Design review of the part built by this model. Coordinates are the model's own, in mm. A direction names the side the tool comes from. Coordinates: 2 decimals unless noted, no trailing zeros. Loops run counter-clockwise (first coordinate to the right, second up) from the corner with the lowest first, then second, coordinate; pieces in that order, holes last. Notation, with made-up numbers: (-5.75, -34) -> (3.25, -34) arc R15 cw to (3.25, -5) -> close; hole circle Ø1 at (71, -36). An arc over 180 degrees is marked (long way). One line per item, written item: value. Start each with the question number.
1. Add section B-B on x = 125.37. Write out the cut boundary in (y, z), plus the area to 3 significant figures.
2. Insertion check: pin 1 (4 mm diameter, centred on x = 7.86, z = 16.83, fed in from -Y). The pin has a flat end and moves straight along its axis. Give the tip position at first contact, or say it passes through.
3. Add section A-A on z = 16.83. Write out the cut boundary in (x, y).
4. Add section C-C on y = 1.15. Write out the cut boundary in (x, z).
5. Add section D-D on x = 80.5. Write out the cut boundary in (y, z).
6. Machinability: for faces 5 (the flat face through (92, 1, 21.85)), 6 (the flat face through (64, 0, 37)), which of the approach directions +Z, -Z, +X, -X, +Y, -Y give a long, thin tool a straight path to every point of the face, cutting with its end or side? Answer none if there is none.
7. For probe 1 along X at (y, z) = (1.4, 22.15); probe 2 along Z at (x, y) = (56.47, 1.25); probe 3 along Z at (x, y) = (95, 1.6), list the stretches that pass through material, from the lowest coordinate up.
8. Draft analysis for pull direction Z (two halves, no side actions). For faces 1 (the flat face through (64, 1, 75.8)), 2 (the flat face through (64, 3, 37)), 3 (the flat face through (119.47, 1, 38)), 4 (the cylindrical face through (8.87, 1.52, 15.72)), state which applies: pulls with the +Z half, pulls with the -Z half, needs draft (parallel to the pull), parting line crosses it, or undercut.
```python
from build123d import *

# Parameters (mm, degrees)
SKETCH1_W           = 130.41
SKETCH1_H           = 75.8
BOSS_EXTRUDE1_DEPTH = 3
SKETCH1_4_W         = 53.3
SKETCH1_4_H         = 32.1
CUT_EXTRUDE2_DEPTH  = 151.868844033
SKETCH1_5_R         = 1.25
CUT_EXTRUDE3_DEPTH  = 151.868844033
SKETCH2_R           = 1.5
CUT_EXTRUDE4_DEPTH  = 151.868844033
SKETCH3_R           = 1.5
CUT_EXTRUDE5_DEPTH  = 151.868844033


with BuildPart() as part:
    # Sketch1 → Boss-Extrude1 (new body)
    with BuildSketch(Plane(origin=(0, 0, 0), x_dir=(1, 0, 0), z_dir=(0, 1, 0))):
        with Locations((65.205, -37.9)):
            Rectangle(SKETCH1_W, SKETCH1_H)
    extrude(amount=BOSS_EXTRUDE1_DEPTH)

    # Sketch1_4 → Cut-Extrude2 (cut, through all)
    with BuildSketch(Plane(origin=(0, 0, 0), x_dir=(1, 0, 0), z_dir=(0, 1, 0))):
        with Locations((92.82, -37.9)):
            Rectangle(SKETCH1_4_W, SKETCH1_4_H)
    extrude(amount=CUT_EXTRUDE2_DEPTH, mode=Mode.SUBTRACT)

    # Sketch1_5 → Cut-Extrude3 (cut, through all)
    with BuildSketch(Plane(origin=(0, 0, 0), x_dir=(1, 0, 0), z_dir=(0, 1, 0))):
        with Locations(Location((56.47, -53.65, 0), (0, 0, 270))):
            Circle(SKETCH1_5_R)
        with Locations(Location((56.47, -22.15, 0), (0, 0, 270))):
            Circle(SKETCH1_5_R)
        with Locations(Location((125.37, -22.15, 0), (0, 0, 270))):
            Circle(SKETCH1_5_R)
        with Locations(Location((125.37, -53.65, 0), (0, 0, 270))):
            Circle(SKETCH1_5_R)
    extrude(amount=CUT_EXTRUDE3_DEPTH, mode=Mode.SUBTRACT)

    # Sketch2 → Cut-Extrude4 (cut, through all)
    with BuildSketch(Plane(origin=(0, 3, 0), x_dir=(1, 0, 0), z_dir=(0, 1, 0))):
        with Locations(Location((7.86, -16.83, 0), (0, 0, 270))):
            Circle(SKETCH2_R)
    extrude(amount=-CUT_EXTRUDE4_DEPTH, mode=Mode.SUBTRACT)

    # Sketch3 → Cut-Extrude5 (cut, through all)
    with BuildSketch(Plane(origin=(0, 3, 0), x_dir=(1, 0, 0), z_dir=(0, 1, 0))):
        with Locations(Location((7.86, -56.71, 0), (0, 0, 270))):
            Circle(SKETCH3_R)
    extrude(amount=-CUT_EXTRUDE5_DEPTH, mode=Mode.SUBTRACT)


solid = part.part
```
Worked answers:
1. outline: (0, 0) -> (3, 0) -> (3, 20.9) -> (0, 20.9) -> close; (0, 23.4) -> (3, 23.4) -> (3, 52.4) -> (0, 52.4) -> close; (0, 54.9) -> (3, 54.9) -> (3, 75.8) -> (0, 75.8) -> close
1. area: 212 mm²
2. pin 1: stops at y = 0
3. outline: (0, 0) -> (6.36, 0) -> (6.36, 3) -> (0, 3) -> close; (9.36, 0) -> (130.41, 0) -> (130.41, 3) -> (9.36, 3) -> close
4. outline: (0, 0) -> (130.41, 0) -> (130.41, 75.8) -> (0, 75.8) -> close; hole circle Ø3 at (7.86, 16.83); hole circle Ø3 at (7.86, 56.71); hole circle Ø2.5 at (56.47, 22.15); hole circle Ø2.5 at (56.47, 53.65); hole (66.17, 21.85) -> (119.47, 21.85) -> (119.47, 53.95) -> (66.17, 53.95) -> close; hole circle Ø2.5 at (125.37, 22.15); hole circle Ø2.5 at (125.37, 53.65)
5. outline: (0, 0) -> (3, 0) -> (3, 21.85) -> (0, 21.85) -> close; (0, 53.95) -> (3, 53.95) -> (3, 75.8) -> (0, 75.8) -> close
6. face 5: +Y, -Y
6. face 6: +Z, -Z, +X, -X, -Y
7. probe 1: x = 0 to 55.22, 57.72 to 66.17, 119.47 to 124.12, 126.62 to 130.41
7. probe 2: z = 0 to 20.9, 23.4 to 52.4, 54.9 to 75.8
7. probe 3: z = 0 to 21.85, 53.95 to 75.8
8. face 1: pulls with the +Z half
8. face 2: needs draft
8. face 3: undercut
8. face 4: undercut
